Job drawing, mm, ordinate dimensions from the low corner. One solid piece. Round coordinates to 2 decimals unless told otherwise and drop trailing zeros. Loops run counter-clockwise (first coordinate to the right, second up) from the corner with the lowest first, then second, coordinate; pieces in that order, holes last. Notation, with made-up numbers: (28.25, 71) - (54.25, 71) arc R20 cw to (54.25, 81) - close; hole circle Ø3 at (79.25, 0). An arc over 180 degrees is marked (long way). Answer as CSV lines item,"result". Start each with the question number.
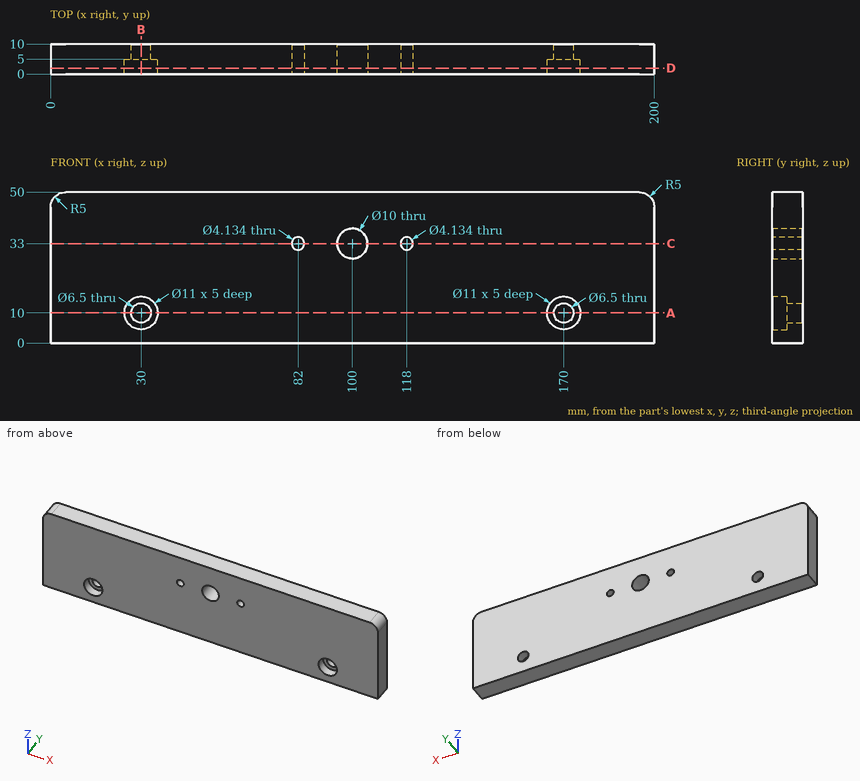
Q1. Band-saw the part on B-B, the plane x = 30. List the corners of the cut face in (y, z).
Q2. Band-saw the part on A-A, the plane z = 10. List the corners of the cut face in (x, y).
Q3. Pin check, flat tips, straight feed: pin 1 Ø6 at (x, z) = (170, 10) entering from -Y; pin 2 Ø5.5 at (x, z) = (29.5, 11) entering from -Y. Stop position of each tip, or through.
Q4. Band-saw the part on D-D, the plane y = 2. List the corners of the cut face in (x, z).
Q5. Band-saw the part on C-C, the plane z = 33. List the corners of the cut face in (x, y), then the cut area to 3 significant figures.
Q6. Wall check: probe 1 along X at (y, z) = (6.45, 10); probe 2 along X at (y, z) = (1.2, 10); probe 3 along X at (y, z) = (5, 33). Give the ranges that are in metal, low to high. Write a range as [from, to].
Reported:
1,outline,"(0, 0) - (10, 0) - (10, 6.75) - (5, 6.75) - (5, 4.5) - (0, 4.5) - close; (0, 15.5) - (5, 15.5) - (5, 13.25) - (10, 13.25) - (10, 50) - (0, 50) - close"
2,outline,"(0, 0) - (24.5, 0) - (24.5, 5) - (26.75, 5) - (26.75, 10) - (0, 10) - close; (33.25, 5) - (35.5, 5) - (35.5, 0) - (164.5, 0) - (164.5, 5) - (166.75, 5) - (166.75, 10) - (33.25, 10) - close; (173.25, 5) - (175.5, 5) - (175.5, 0) - (200, 0) - (200, 10) - (173.25, 10) - close"
3,pin 1,"passes through"
3,pin 2,"stops at y = 5"
4,outline,"(0, 0) - (200, 0) - (200, 45) arc R5 ccw to (195, 50) - (5, 50) arc R5 ccw to (0, 45) - close; hole circle Ø11 at (30, 10); hole circle Ø4.13 at (82, 33); hole circle Ø10 at (100, 33); hole circle Ø4.13 at (118, 33); hole circle Ø11 at (170, 10)"
5,outline,"(0, 0) - (79.93, 0) - (79.93, 10) - (0, 10) - close; (84.07, 0) - (95, 0) - (95, 10) - (84.07, 10) - close; (105, 0) - (115.93, 0) - (115.93, 10) - (105, 10) - close; (120.07, 0) - (200, 0) - (200, 10) - (120.07, 10) - close"
5,area,"1,820 mm2"
6,probe 1,"x = [0, 26.75], [33.25, 166.75], [173.25, 200]"
6,probe 2,"x = [0, 24.5], [35.5, 164.5], [175.5, 200]"
6,probe 3,"x = [0, 79.93], [84.07, 95], [105, 115.93], [120.07, 200]"
